Job drawing, mm, ordinate dimensions from the low corner. One solid piece. A direction names the side the tool comes from. Round coordinates to 2 decimals unless told otherwise and drop trailing zeros. Order: outer loops, then holes, each group sorted by start corner. A loop starts at its lowest first (then second) coordinate and runs counter-clockwise, first axis right, second up. Notation, with made-up numbers: (-24.5, 65) -> (32.5, 65) arc R8 ccw to (32.5, 71) -> close; hole circle Ø7 at (19.5, 47.25). An arc over 180 degrees is marked (long way). Return JSON: item names as keys, results as strings. Group by question number.
Q1. Cut at A-A (z = 85). Write the cut outline in (x, y).
Q2. Flat gauge pins, fed straight in: pin 1 (10 mm diameter, centred on x = 60, z = 6.5, fed in from -Y); pin 2 (4.5 mm diameter, centred on x = 65.5, y = 11.5, fed in from -Z); pin 3 (1.5 mm diameter, centred on y = 24.5, z = 12.5, fed in from -X); pin 4 (1 mm diameter, centred on x = 59, z = 78, fed in from -Y). Where does each tip first touch, or does it go through?
Q3. Probe line 1 along X through (y, z) = (26, 25); line 2 along Y through (x, z) = (71, 67); line 3 along Z through (x, y) = (49, 19). List the from-to ranges inside material, lowest first.
Q4. Which spindle directions (+Z, -Z, +X, -X, +Y, -Y) get a long thin tool onto all of the face, cutting with end or side? Do the marked faces 1, 2, 3 and 4. Say none if no direction does.
Q5. Cut at C-C (z = 46). Write the cut outline in (x, y), then the cut area to 3 significant figures.
Q6. Mould opens along Y. For the marked faces 5, 6, 7 and 8 say: +Y half, -Y half, draft (parallel to the pull), parting line (faces both ways), or undercut.
Q7. Cut at B-B (y = 5.5). Write the cut outline in (x, z) (1 decimal), then the cut area to 3 significant figures.
Q8. Cut at D-D (x = 54). Write the cut outline in (y, z), then the cut area to 3 significant figures.
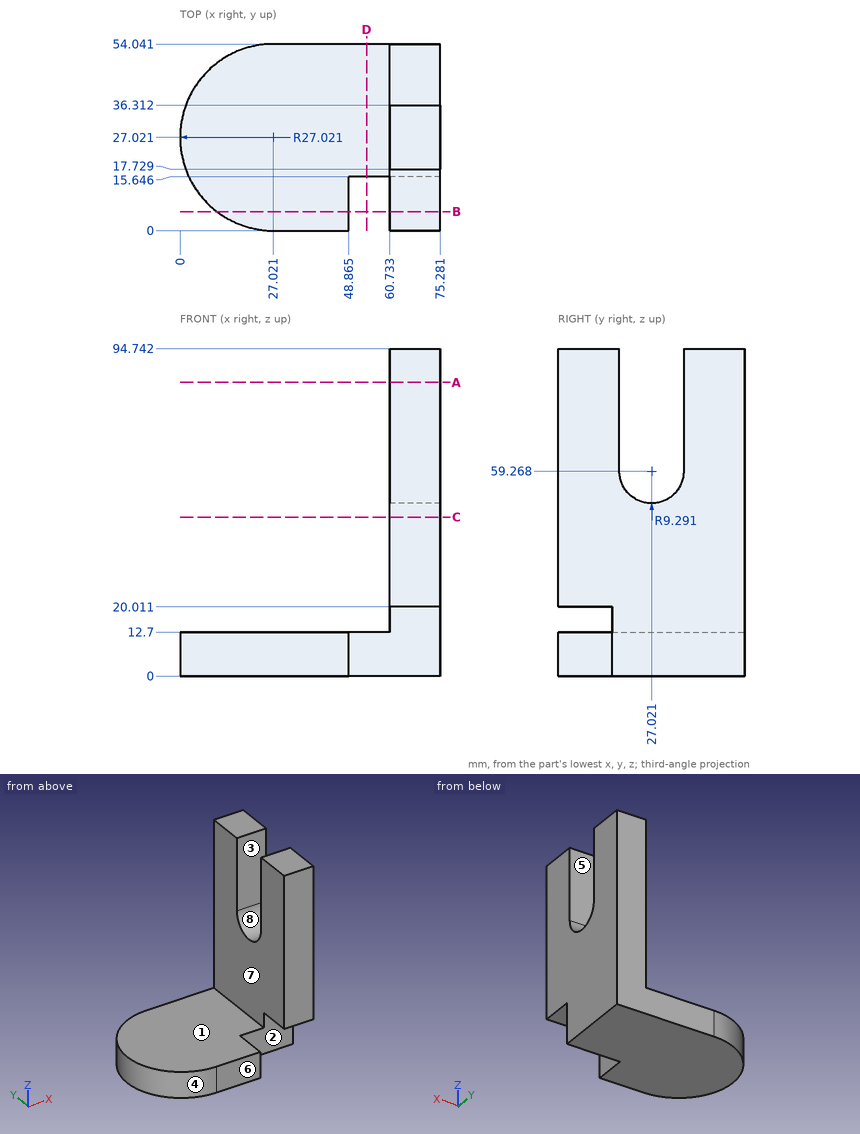
Solution:
{
 "1": {"outline": "(60.73, 0) -> (75.28, 0) -> (75.28, 17.73) -> (60.73, 17.73) -> close; (60.73, 36.31) -> (75.28, 36.31) -> (75.28, 54.04) -> (60.73, 54.04) -> close"},
 "2": {"pin 1": "stops at y = 15.65", "pin 2": "stops at z = 20.01", "pin 3": "stops at x = 0.06", "pin 4": "passes through"},
 "3": {"line 1": "x = 60.73 to 75.28", "line 2": "y = 0 to 17.73, 36.31 to 54.04", "line 3": "z = 0 to 12.7"},
 "4": {"face 1": "+Z, -X, +Y, -Y", "face 2": "-Z, +X, -Y", "face 3": "+Z, +X, -X", "face 4": "+Z, -Z, -X"},
 "5": {"outline": "(60.73, 0) -> (75.28, 0) -> (75.28, 54.04) -> (60.73, 54.04) -> close", "area": "786 mm²"},
 "6": {"face 5": "undercut", "face 6": "-Y half", "face 7": "draft", "face 8": "undercut"},
 "7": {"outline": "(10.7, 0) -> (48.9, 0) -> (48.9, 12.7) -> (10.7, 12.7) -> close; (60.7, 20) -> (75.3, 20) -> (75.3, 94.7) -> (60.7, 94.7) -> close", "area": "1,570 mm²"},
 "8": {"outline": "(15.65, 0) -> (54.04, 0) -> (54.04, 12.7) -> (15.65, 12.7) -> close", "area": "488 mm²"}
}
